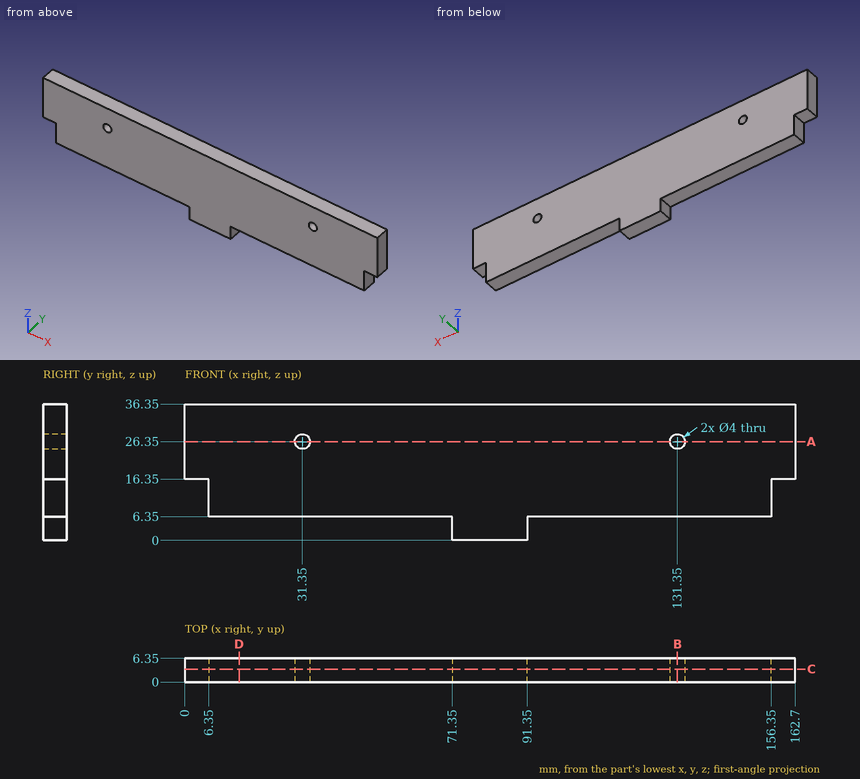
The drawing under review shows one solid part. Ordinate dimensions are in mm from its lowest x, y, z. Round coordinates to 2 decimals unless told otherwise and drop trailing zeros. Loops run counter-clockwise (first coordinate to the right, second up) from the corner with the lowest first, then second, coordinate; pieces in that order, holes last. Notation, with made-up numbers: (76.25, -27.5) -> (95.25, -27.5) arc R12 ccw to (95.25, -7.5) -> close; hole circle Ø1 at (37.5, 49). An arc over 180 degrees is marked (long way). Answer in a Markdown table with one row per item.
1) Consider section A-A, the plane z = 26.35. Write out the cut boundary in (x, y), plus the area to 3 significant figures.
Taken from the geometry:
| item | result |
|---|---|
| outline | (0, 0) -> (29.35, 0) -> (29.35, 6.35) -> (0, 6.35) -> close; (33.35, 0) -> (129.35, 0) -> (129.35, 6.35) -> (33.35, 6.35) -> close; (133.35, 0) -> (162.7, 0) -> (162.7, 6.35) -> (133.35, 6.35) -> close |
| area | 982 mm² |
2) Consider section D-D, the plane x = 14.5. Write out the cut boundary in (y, z).
Taken from the geometry:
| item | result |
|---|---|
| outline | (0, 6.35) -> (6.35, 6.35) -> (6.35, 36.35) -> (0, 36.35) -> close |
3) For pin 1 Ø3 at (y, z) = (2, 4) entering from +X; pin 2 Ø1.9 at (y, z) = (4, 11) entering from -X; pin 3 Ø3 at (y, z) = (4, 10) entering from +X, all flat-tipped, find the tip position at first contact; note any pin that passes through.
Taken from the geometry:
| item | result |
|---|---|
| pin 1 | stops at x = 91.35 |
| pin 2 | stops at x = 6.35 |
| pin 3 | stops at x = 156.35 |
4) Consider section C-C, the plane y = 3.5. Write out the cut boundary in (x, z).
Taken from the geometry:
| item | result |
|---|---|
| outline | (0, 16.35) -> (6.35, 16.35) -> (6.35, 6.35) -> (71.35, 6.35) -> (71.35, 0) -> (91.35, 0) -> (91.35, 6.35) -> (156.35, 6.35) -> (156.35, 16.35) -> (162.7, 16.35) -> (162.7, 36.35) -> (0, 36.35) -> close; hole circle Ø4 at (31.35, 26.35); hole circle Ø4 at (131.35, 26.35) |
5) Consider section B-B, the plane x = 131.35. Write out the cut boundary in (y, z).
Taken from the geometry:
| item | result |
|---|---|
| outline | (0, 6.35) -> (6.35, 6.35) -> (6.35, 24.35) -> (0, 24.35) -> close; (0, 28.35) -> (6.35, 28.35) -> (6.35, 36.35) -> (0, 36.35) -> close |
6) Wall thickness on line 1 along X through (y, z) = (2.5, 26.35); line 2 along X through (y, z) = (5, 28); line 3 along Z through (x, y) = (152.5, 4.75): over which ranges is each line inside the solid? List them lowest first.
Taken from the geometry:
| item | result |
|---|---|
| line 1 | x = 0 to 29.35, 33.35 to 129.35, 133.35 to 162.7 |
| line 2 | x = 0 to 30.22, 32.48 to 130.22, 132.48 to 162.7 |
| line 3 | z = 6.35 to 36.35 |
